Can you work these out from the model? Positions are in its coordinate system, mm. A direction names the side the tool comes from. Round coordinates to 2 decimals unless told otherwise and drop trailing zeros. Write each loop counter-clockwise with the first axis right and the second up, starting at its lowest first coordinate (ties: lowest second). Pieces come first, ordered by that corner, then holes. Notation, with made-up numbers: (39.25, 76) -> (94.25, 76) arc R9 cw to (94.25, 93) -> close; hole circle Ø7 at (20, 79.5). An arc over 180 degrees is marked (long way). Use CSV: the item, a comma, the result in double quotes.
```python
from build123d import *

# Parameters (mm, degrees)
SKETCH1_R                        = 4
SKETCH1_R_2                      = 1.75
BOSS_EXTRUDE1_DEPTH              = 3
SKETCH2_R                        = 4
SKETCH2_R_2                      = 3
BOSS_EXTRUDE2_DEPTH              = 2.5
TAP_DRILL_FOR_M2X0_4_TAP1_REACH  = 11.852
TAP_DRILL_FOR_M2X0_4_TAP1_BORE_R = 0.8


with BuildPart() as part:
    # Sketch1 → Boss-Extrude1 (new body)
    with BuildSketch(Plane.XY):
        Circle(SKETCH1_R)
        Circle(SKETCH1_R_2, mode=Mode.SUBTRACT)
    extrude(amount=BOSS_EXTRUDE1_DEPTH)

    # Sketch2 → Boss-Extrude2 (add)
    with BuildSketch(Plane.XY.offset(3)):
        Circle(SKETCH2_R)
        Circle(SKETCH2_R_2, mode=Mode.SUBTRACT)
    extrude(amount=BOSS_EXTRUDE2_DEPTH)

    # Tap Drill for M2x0.4 Tap1 bore (on position points) → Tap Drill for M2x0.4 Tap1 (cut, up to next)
    with BuildSketch(Plane(origin=(0.135818607, -3.997693498, 1.5), x_dir=(-0.999423374561, -0.033954651826, 0), z_dir=(0.033954651826, -0.999423374561, 0)), mode=Mode.PRIVATE) as tap_drill_for_m2x0_4_tap1_sk1:
        Circle(TAP_DRILL_FOR_M2X0_4_TAP1_BORE_R)
    tap_drill_for_m2x0_4_tap1_tool1 = extrude(tap_drill_for_m2x0_4_tap1_sk1.sketch, amount=-TAP_DRILL_FOR_M2X0_4_TAP1_REACH, mode=Mode.PRIVATE) & part.part
    add(tap_drill_for_m2x0_4_tap1_tool1.solids().sort_by_distance((0.135819, -3.997693, 1.5))[0], mode=Mode.SUBTRACT)


solid = part.part
```
Q1. Suppose I cut it at C-C (x = 0). Count the separate pieces of the cut face and the enclosed holes in it, and give its area (3 significant figures).
Resolved:
separate pieces,"3"
enclosed holes,"0"
area,"14.9 mm^2"
Q2. Suppose I cut it at D-D (x = 2.75). Write out the boundary of the cut face in (y, z), and give its area (3 significant figures).
Resolved:
outline,"(-2.9, 0) -> (2.9, 0) -> (2.9, 5.5) -> (1.2, 5.5) -> (1.2, 3) -> (-1.2, 3) -> (-1.2, 5.5) -> (-2.9, 5.5) -> close"
area,"26.0 mm^2"
Q3. Will these pins go through, and if not, where does the flat tip stop? P1, Ø3, axis at y = -3, z = 3.5, coming from the +X side; P2, Ø2, axis at x = 2, z = 1, coming from the +Y side.
Resolved:
P1,"stops at x = 3.71"
P2,"stops at y = 3.87"
Q4. If we mould it in two halves opening along Y, with no side actions, what happens to faces 3 (the face through (-0.867, -3.905, 2.712)), 4 (the face through (0.199, -2.79, 0.707)), 5 (the face through (1, 3, 5.5))? For each: released by +Y, released by -Y, zero draft, split by the parting line, or undercut.
Resolved:
face 3,"split by the parting line"
face 4,"undercut"
face 5,"zero draft"
Q5. Please list where these lines run through material, in increasing order: probe 1 along Y at (x, z) = (0, 3.5); probe 2 along Z at (x, y) = (-1.75, -0.75); probe 3 along Y at (x, z) = (0, 2.15).
Resolved:
probe 1,"y = -4 to -3, 3 to 4"
probe 2,"z = 0 to 3"
probe 3,"y = 1.75 to 4"
Q6. Suppose I cut it at A-A (y = 0). Write out the boundary of the cut face in (x, z), and give its area (3 significant figures).
Resolved:
outline,"(-4, 0) -> (-1.75, 0) -> (-1.75, 3) -> (-3, 3) -> (-3, 5.5) -> (-4, 5.5) -> close; (1.75, 0) -> (4, 0) -> (4, 5.5) -> (3, 5.5) -> (3, 3) -> (1.75, 3) -> close"
area,"18.5 mm^2"
Q7. On a 3-axis mill with a long thin cutter (end or side, diameter ignored), from which of +Z, -Z, +X, -X, +Y, -Y can I reach the whole of each face in a straight line? I mean faces 1 (the face through (-0.228, 1.735, 1.479)), 2 (the face through (-3, 0, 4)). Say none if no direction works.
Resolved:
face 1,"+Z, -Z"
face 2,"+Z"
Q8. Suppose I cut it at B-B (z = 4.1). Write out the boundary of the cut face in (x, y).
Resolved:
outline,"circle Ø8 at (0, 0); hole circle Ø6 at (0, 0)"
